```python
from build123d import *

# Parameters (mm, degrees)
F1_DEPTH = 2
F3_DEPTH = 25
F5_DEPTH = 2


with BuildPart() as f1:
    # F0 (on Top) → F1 (new body)
    with BuildSketch(Plane.XY):
        with BuildLine():
            ThreePointArc((36.403983, -9), (32.451992, -3.951992), (37.5, 0))
            ThreePointArc((37.5, 0), (37.394112, 2.816094), (37.077046, 5.616285))
            ThreePointArc((37.077046, 5.616285), (31.494093, 8.767675), (34.645482, 14.350629))
            ThreePointArc((34.645482, 14.350629), (33.469982, 16.911839), (32.105464, 19.377542))
            ThreePointArc((32.105464, 19.377542), (25.741503, 20.152543), (26.516504, 26.516504))
            ThreePointArc((26.516504, 26.516504), (24.450351, 28.43291), (22.246117, 30.188744))
            ThreePointArc((22.246117, 30.188744), (16.070004, 28.469369), (14.350629, 34.645482))
            ThreePointArc((14.350629, 34.645482), (11.708375, 35.625327), (9, 36.403983))
            ThreePointArc((9, 36.403983), (3.951992, 32.451992), (0, 37.5))
            ThreePointArc((0, 37.5), (-2.816094, 37.394112), (-5.616285, 37.077046))
            ThreePointArc((-5.616285, 37.077046), (-8.767675, 31.494093), (-14.350629, 34.645482))
            ThreePointArc((-14.350629, 34.645482), (-16.911839, 33.469982), (-19.377542, 32.105464))
            ThreePointArc((-19.377542, 32.105464), (-20.152543, 25.741503), (-26.516504, 26.516504))
            ThreePointArc((-26.516504, 26.516504), (-28.43291, 24.450351), (-30.188744, 22.246117))
            ThreePointArc((-30.188744, 22.246117), (-28.469369, 16.070004), (-34.645482, 14.350629))
            ThreePointArc((-34.645482, 14.350629), (-35.625327, 11.708375), (-36.403983, 9))
            ThreePointArc((-36.403983, 9), (-32.451992, 3.951992), (-37.5, 0))
            ThreePointArc((-37.5, 0), (-37.394112, -2.816094), (-37.077046, -5.616285))
            ThreePointArc((-37.077046, -5.616285), (-31.494093, -8.767675), (-34.645482, -14.350629))
            ThreePointArc((-34.645482, -14.350629), (-33.469982, -16.911839), (-32.105464, -19.377542))
            ThreePointArc((-32.105464, -19.377542), (-25.741503, -20.152543), (-26.516504, -26.516504))
            ThreePointArc((-26.516504, -26.516504), (-24.450351, -28.43291), (-22.246117, -30.188744))
            ThreePointArc((-22.246117, -30.188744), (-16.070004, -28.469369), (-14.350629, -34.645482))
            ThreePointArc((-14.350629, -34.645482), (-11.708375, -35.625327), (-9, -36.403983))
            ThreePointArc((-9, -36.403983), (-3.951992, -32.451992), (0, -37.5))
            ThreePointArc((0, -37.5), (2.816094, -37.394112), (5.616285, -37.077046))
            ThreePointArc((5.616285, -37.077046), (8.767675, -31.494093), (14.350629, -34.645482))
            ThreePointArc((14.350629, -34.645482), (16.911839, -33.469982), (19.377542, -32.105464))
            ThreePointArc((19.377542, -32.105464), (20.152543, -25.741503), (26.516504, -26.516504))
            ThreePointArc((26.516504, -26.516504), (28.43291, -24.450351), (30.188744, -22.246117))
            ThreePointArc((30.188744, -22.246117), (28.469369, -16.070004), (34.645482, -14.350629))
            ThreePointArc((34.645482, -14.350629), (35.625327, -11.708375), (36.403983, -9))
        make_face()
    extrude(amount=F1_DEPTH)

    # F2 (on face) → F3 (cut)
    with BuildSketch(Plane.XY.offset(2)):
        with BuildLine():
            ThreePointArc((-20, 0), (-18.477591, 7.653669), (-14.142136, 14.142136))
            ThreePointArc((-14.142136, 14.142136), (-14.142136, 21.213203), (-21.213203, 21.213203))
            ThreePointArc((-21.213203, 21.213203), (-27.716386, 11.480503), (-30, 0))
            ThreePointArc((-30, 0), (-25, -5), (-20, 0))
        make_face()
        with BuildLine():
            ThreePointArc((0, 20), (7.653669, 18.477591), (14.142136, 14.142136))
            ThreePointArc((14.142136, 14.142136), (21.213203, 14.142136), (21.213203, 21.213203))
            ThreePointArc((21.213203, 21.213203), (11.480503, 27.716386), (0, 30))
            ThreePointArc((0, 30), (-5, 25), (0, 20))
        make_face()
        with BuildLine():
            ThreePointArc((20, 0), (18.477591, -7.653669), (14.142136, -14.142136))
            ThreePointArc((14.142136, -14.142136), (14.142136, -21.213203), (21.213203, -21.213203))
            ThreePointArc((21.213203, -21.213203), (27.716386, -11.480503), (30, 0))
            ThreePointArc((30, 0), (25, 5), (20, 0))
        make_face()
        with BuildLine():
            ThreePointArc((0, -20), (-7.653669, -18.477591), (-14.142136, -14.142136))
            ThreePointArc((-14.142136, -14.142136), (-21.213203, -14.142136), (-21.213203, -21.213203))
            ThreePointArc((-21.213203, -21.213203), (-11.480503, -27.716386), (0, -30))
            ThreePointArc((0, -30), (5, -25), (0, -20))
        make_face()
    extrude(amount=-F3_DEPTH, mode=Mode.SUBTRACT)

    # F4 (on face) → F5 (cut)
    with BuildSketch(Plane.XY.offset(2)):
        with BuildLine():
            Line((8.427281, 1.109473), (9.914449, 1.305262))
            ThreePointArc((9.914449, 1.305262), (9.490349, 3.151709), (8.72562, 4.885034))
            Line((8.72562, 4.885034), (7.416777, 4.152279))
            ThreePointArc((7.416777, 4.152279), (7.098564, 4.67551), (6.743503, 5.174472))
            Line((6.743503, 5.174472), (7.933533, 6.087614))
            ThreePointArc((7.933533, 6.087614), (6.643029, 7.474635), (5.114091, 8.593374))
            Line((5.114091, 8.593374), (4.346978, 7.304368))
            ThreePointArc((4.346978, 7.304368), (3.809781, 7.598392), (3.252809, 7.852976))
            Line((3.252809, 7.852976), (3.826834, 9.238795))
            ThreePointArc((3.826834, 9.238795), (2.015715, 9.794738), (0.132246, 9.999126))
            Line((0.132246, 9.999126), (0.112409, 8.499257))
            ThreePointArc((0.112409, 8.499257), (-0.499829, 8.485291), (-1.109473, 8.427281))
            Line((-1.109473, 8.427281), (-1.305262, 9.914449))
            ThreePointArc((-1.305262, 9.914449), (-3.151709, 9.490349), (-4.885034, 8.72562))
            Line((-4.885034, 8.72562), (-4.152279, 7.416777))
            ThreePointArc((-4.152279, 7.416777), (-4.67551, 7.098564), (-5.174472, 6.743503))
            Line((-5.174472, 6.743503), (-6.087614, 7.933533))
            ThreePointArc((-6.087614, 7.933533), (-7.474635, 6.643029), (-8.593374, 5.114091))
            Line((-8.593374, 5.114091), (-7.304368, 4.346978))
            ThreePointArc((-7.304368, 4.346978), (-7.598392, 3.809781), (-7.852976, 3.252809))
            Line((-7.852976, 3.252809), (-9.238795, 3.826834))
            ThreePointArc((-9.238795, 3.826834), (-9.794738, 2.015715), (-9.999126, 0.132246))
            Line((-9.999126, 0.132246), (-8.499257, 0.112409))
            ThreePointArc((-8.499257, 0.112409), (-8.485291, -0.499829), (-8.427281, -1.109473))
            Line((-8.427281, -1.109473), (-9.914449, -1.305262))
            ThreePointArc((-9.914449, -1.305262), (-9.490349, -3.151709), (-8.72562, -4.885034))
            Line((-8.72562, -4.885034), (-7.416777, -4.152279))
            ThreePointArc((-7.416777, -4.152279), (-7.098564, -4.67551), (-6.743503, -5.174472))
            Line((-6.743503, -5.174472), (-7.933533, -6.087614))
            ThreePointArc((-7.933533, -6.087614), (-6.643029, -7.474635), (-5.114091, -8.593374))
            Line((-5.114091, -8.593374), (-4.346978, -7.304368))
            ThreePointArc((-4.346978, -7.304368), (-3.809781, -7.598392), (-3.252809, -7.852976))
            Line((-3.252809, -7.852976), (-3.826834, -9.238795))
            ThreePointArc((-3.826834, -9.238795), (-2.015715, -9.794738), (-0.132246, -9.999126))
            Line((-0.132246, -9.999126), (-0.112409, -8.499257))
            ThreePointArc((-0.112409, -8.499257), (0.499829, -8.485291), (1.109473, -8.427281))
            Line((1.109473, -8.427281), (1.305262, -9.914449))
            ThreePointArc((1.305262, -9.914449), (3.151709, -9.490349), (4.885034, -8.72562))
            Line((4.885034, -8.72562), (4.152279, -7.416777))
            ThreePointArc((4.152279, -7.416777), (4.67551, -7.098564), (5.174472, -6.743503))
            Line((5.174472, -6.743503), (6.087614, -7.933533))
            ThreePointArc((6.087614, -7.933533), (7.474635, -6.643029), (8.593374, -5.114091))
            Line((8.593374, -5.114091), (7.304368, -4.346978))
            ThreePointArc((7.304368, -4.346978), (7.598392, -3.809781), (7.852976, -3.252809))
            Line((7.852976, -3.252809), (9.238795, -3.826834))
            ThreePointArc((9.238795, -3.826834), (9.794738, -2.015715), (9.999126, -0.132246))
            Line((9.999126, -0.132246), (8.499257, -0.112409))
            ThreePointArc((8.499257, -0.112409), (8.485291, 0.499829), (8.427281, 1.109473))
        make_face()
    extrude(amount=-F5_DEPTH, mode=Mode.SUBTRACT)


solid = f1.part
```
For this review, take the finished solid that the model builds, in its own axes (mm). A direction names the side the tool comes from. Give positions to 0.01 mm unless a question says otherwise; leave off trailing zeros. Write each loop counter-clockwise with the first axis right and the second up, starting at its lowest first coordinate (ties: lowest second). Pieces come first, ordered by that corner, then holes. Notation, with made-up numbers: M 81.25,9.5 L 85.25,9.5 A29 cw 85.25,35.5 Z; hole C 5.5,-24 d1. An arc over 180 degrees is marked long. Answer as a JSON object with one key per item and string values. Group by question number.
Item 1: Consider section C-C on x = 11.5. Write out the cut boundary in (y, z).
Item 2: Draft analysis for pull direction Y (two halves, no side actions). For faces 3 (the cylindrical face through (-28.4, 16.2, 1)), 4 (the cylindrical face through (-11.75, -35.61, 0.99)), 5 (the cylindrical face through (-18.5, 7.6, 1)), 6 (the cylindrical face through (-35.61, 11.75, 0.99)), state which applies: +Y half, -Y half, draft (parallel to the pull), parting line (faces both ways), or undercut.
Item 3: Tool access review of faces 1 (the cylindrical face through (-28.41, 24.48, 0.99)), 2 (the cylindrical face through (5, -25, 1)): name each direction out of +Z, -Z, +X, -X, +Y, -Y from which nothing blocks a thin tool from reaching the whole face with its end or side.
Item 4: For probe 1 along X at (y, z) = (-17.5, 0.55); probe 2 along X at (y, z) = (34.5, 0.9); probe 3 along Y at (x, z) = (8, 0.7), list the stretches that pass through material, from the lowest coordinate up. Write a range as [from, to].
Item 5: Consider section A-A on y = 16.5. Write out the cut boundary in (x, z).
Item 6: Consider section D-D on y = -16. Write out the cut boundary in (x, z).
Item 7: Consider section B-B on z = 1. Count the separate pieces of the cut face and the enclosed holes in it, plus the area to 3 significant figures.
Item 8: For pin 1 Ø1 at (x, z) = (11.5, 1.5) entering from -Y, flat-tipped, find the tip position at first contact; note if it passes through.
Check result:
{
 "1": {"outline": "M -31.59,0 L 16.36,0 L 16.36,2 L -31.59,2 Z; M 27.71,0 L 35.69,0 L 35.69,2 L 27.71,2 Z"},
 "2": {"face 3": "undercut", "face 4": "-Y half", "face 5": "undercut", "face 6": "+Y half"},
 "3": {"face 1": "+Z, -Z, -X, +Y", "face 2": "+Z, -Z"},
 "4": {"probe 1": "x = [-33.17, -22.67], [-9.68, 12.68], [24.37, 27.95]", "probe 2": "x = [-14.7, -14.31], [-5.66, 0.69], [8.31, 14.27]", "probe 3": "y = [-31.78, -6], [-4.76, -3.31], [4.48, 18.33], [28.91, 34.07]"},
 "5": {"outline": "M -28.26,0 L -25.05,0 L -25.05,2 L -28.26,2 Z; M -12.82,0 L 11.3,0 L 11.3,2 L -12.82,2 Z; M 22.54,0 L 33.67,0 L 33.67,2 L 22.54,2 Z"},
 "6": {"outline": "M -33.92,0 L -22.39,0 L -22.39,2 L -33.92,2 Z; M -12,0 L 12.97,0 L 12.97,2 L -12,2 Z; M 25.38,0 L 28.51,0 L 28.51,2 L 25.38,2 Z"},
 "7": {"separate pieces": "1", "enclosed holes": "5", "area": "2,490 mm^2"},
 "8": {"pin 1": "stops at y = -31.8"}
}
